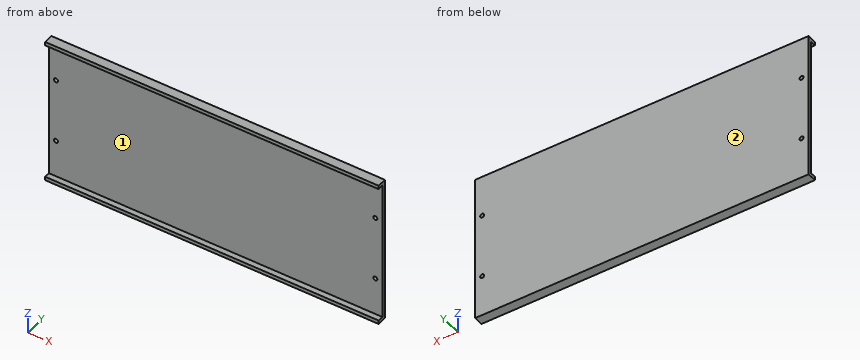
from build123d import *

# Parameters (mm, degrees)
SKETCH_1_W      = 179.6
SKETCH_1_H      = 76
SKETCH_1_R      = 1.1
EXTRUDE_1_DEPTH = 2
SKETCH_2_W      = 179.6
SKETCH_2_H      = 2
EXTRUDE_2_DEPTH = 5


with BuildPart() as part:
    # 草图1 → 凸台-拉伸1 (new body)
    with BuildSketch(Plane(origin=(0, 0, 0), x_dir=(1, 0, 0), z_dir=(0, 1, 0))):
        Rectangle(SKETCH_1_W, SKETCH_1_H)
        with Locations(Location((-86, 17.5, 0), (0, 0, 270))):
            Circle(SKETCH_1_R, mode=Mode.SUBTRACT)
        with Locations(Location((-86, -17.5, 0), (0, 0, 90))):
            Circle(SKETCH_1_R, mode=Mode.SUBTRACT)
        with Locations(Location((86, -17.5, 0), (0, 0, 270))):
            Circle(SKETCH_1_R, mode=Mode.SUBTRACT)
        with Locations(Location((86, 17.5, 0), (0, 0, 90))):
            Circle(SKETCH_1_R, mode=Mode.SUBTRACT)
    extrude(amount=EXTRUDE_1_DEPTH)

    # 草图2 → 凸台-拉伸2 (add)
    with BuildSketch(Plane(origin=(0, 2, 0), x_dir=(1, 0, 0), z_dir=(0, 1, 0))):
        with Locations((0, 39)):
            Rectangle(SKETCH_2_W, SKETCH_2_H)
        with Locations((0, -39)):
            Rectangle(SKETCH_2_W, SKETCH_2_H)
    extrude(amount=-EXTRUDE_2_DEPTH)


solid = part.part
Read the model definition and answer for the solid it produces. Units are mm, in the model's axes. Face numbers are marked on the shaded views. Coordinates: 2 decimals unless noted, no trailing zeros. Loops run counter-clockwise (first coordinate to the right, second up) from the corner with the lowest first, then second, coordinate; pieces in that order, holes last.
Q1. Consider probe 1 along Z at (x, y) = (-86, 0.8); probe 2 along X at (y, z) = (1.6, 17.5); probe 3 along Z at (x, y) = (-10.5, -1.15). Determine where each line is inside the solid, lowest interval first.
Q2. The part is cut by section C-C on z = 10. Write down the section's boundary in (x, y), and give its area (3 significant figures).
Q3. This flat-tipped pin is pushed along its axis until it touches: pin 1 Ø4 at (x, z) = (-40.5, -26) entering from -Y. Where does it stop, or does it pass through?
Q4. The part is cut by section B-B on x = -74.5. Write down the section's boundary in (y, z), and give its area (3 significant figures).
Q5. The part is cut by section A-A on y = -1.15. Write down the section's boundary in (x, z).
Q6. The mould has two halves that part along Z. Classify the marked faces 1 and 2: +Z half, -Z half, draft (parallel to the pull), parting line (faces both ways), or undercut.
Results below:
1. probe 1: z = -40 to -18.6, -16.4 to 16.4, 18.6 to 40
1. probe 2: x = -89.8 to -87.1, -84.9 to 84.9, 87.1 to 89.8
1. probe 3: z = -40 to -38, 38 to 40
2. outline: (-89.8, 0) - (89.8, 0) - (89.8, 2) - (-89.8, 2) - close
2. area: 359 mm2
3. pin 1: stops at y = 0
4. outline: (-3, -40) - (2, -40) - (2, 40) - (-3, 40) - (-3, 38) - (0, 38) - (0, -38) - (-3, -38) - close
4. area: 172 mm2
5. outline: (-89.8, -40) - (89.8, -40) - (89.8, -38) - (-89.8, -38) - close; (-89.8, 38) - (89.8, 38) - (89.8, 40) - (-89.8, 40) - close
6. face 1: undercut
6. face 2: draft
